Geometry check sheet. Reference: the model listing, model coordinates, mm. Round coordinates to 2 decimals unless told otherwise and drop trailing zeros. Write each loop counter-clockwise with the first axis right and the second up, starting at its lowest first coordinate (ties: lowest second). Pieces come first, ordered by that corner, then holes. Notation, with made-up numbers: M -6,24 L 35,24 A10 ccw 35,43 Z; hole C 24,39 d8. An arc over 180 degrees is marked long. Put each result on its own line as item: value. Start each with the question number.
(1) Material ranges on probe 1 along X at (y, z) = (6, 0); probe 2 along X at (y, z) = (4.5, -86); probe 3 along Z at (x, y) = (83.5, 5.5), recorded low to high.
(2) Mould release check, pull along Z, two halves, no side actions. Record for faces 1 (the cylindrical face through (0, 5, 82)), 2 (the flat face through (-2, 5, -150)), 3 (the flat face through (150, 5, 2)): pulls with the +Z half, pulls with the -Z half, needs draft (parallel to the pull), parting line crosses it, or undercut.
(3) Gauge pin test, flat end, axial feed: pin 1 (5 mm diameter, centred on x = 0, z = 86, fed in from -Y). Record the tip position at first contact, or that the pin passes through.
(4) Section check B-B on z = 86. Record the cut outline in (x, y), then the cut area to 3 significant figures.
(5) Section check A-A on x = 0. Record the cut outline in (y, z), then the cut area to 3 significant figures.
(6) Section check C-C on z = 0. Record the cut outline in (x, y), then the cut area to 3 significant figures.
from build123d import *

# Parameters (mm, degrees)
SKETCH_1_W          = 300
SKETCH_1_H          = 300
EXTRUDE_1_DEPTH     = 10
CHAMFER_1_SIZE      = 5
SKETCH_2_R          = 4
CUT_EXTRUDE_1_DEPTH = 10


with BuildPart() as part:
    # 스케치1 → 보스-돌출1 (new body)
    with BuildSketch(Plane(origin=(0, 0, 0), x_dir=(1, 0, 0), z_dir=(0, 1, 0))):
        Rectangle(SKETCH_1_W, SKETCH_1_H)
    extrude(amount=EXTRUDE_1_DEPTH)

    # 모따기1
    chamfer_1_edges = [part.edges().sort_by_distance(p)[0] for p in [
        (150, 5, 150),
        (-150, 5, 150),
        (-150, 5, -150),
        (150, 5, -150),
    ]]
    chamfer(chamfer_1_edges, length=CHAMFER_1_SIZE)

    # 스케치2 → 컷-돌출1 (cut)
    with BuildSketch(Plane(origin=(0, 10, 0), x_dir=(1, 0, 0), z_dir=(0, 1, 0))):
        with Locations(Location((0, -86, 0), (0, 0, 270))):
            Circle(SKETCH_2_R)
        with Locations(Location((-86, 0, 0), (0, 0, 270))):
            Circle(SKETCH_2_R)
        with Locations(Location((0, 86, 0), (0, 0, 270))):
            Circle(SKETCH_2_R)
        with Locations(Location((86, 0, 0), (0, 0, 270))):
            Circle(SKETCH_2_R)
    extrude(amount=-CUT_EXTRUDE_1_DEPTH, mode=Mode.SUBTRACT)


solid = part.part
Answers follow:
1. probe 1: x = -150 to -90, -82 to 82, 90 to 150
1. probe 2: x = -150 to -4, 4 to 150
1. probe 3: z = -150 to -3.12, 3.12 to 150
2. face 1: undercut
2. face 2: pulls with the -Z half
2. face 3: needs draft
3. pin 1: passes through
4. outline: M -150,0 L -4,0 L -4,10 L -150,10 Z; M 4,0 L 150,0 L 150,10 L 4,10 Z
4. area: 2,920 mm^2
5. outline: M 0,-150 L 10,-150 L 10,-90 L 0,-90 Z; M 0,-82 L 10,-82 L 10,82 L 0,82 Z; M 0,90 L 10,90 L 10,150 L 0,150 Z
5. area: 2,840 mm^2
6. outline: M -150,0 L -90,0 L -90,10 L -150,10 Z; M -82,0 L 82,0 L 82,10 L -82,10 Z; M 90,0 L 150,0 L 150,10 L 90,10 Z
6. area: 2,840 mm^2
